```python
from build123d import *

# Parameters (mm, degrees)
F0_W         = 8.5
F0_H         = 13.5
F0_W_2       = 1.7211329822
F0_H_2       = 1.5
F0_W_3       = 1.7788670178
F1_DEPTH     = 0.9
F2_DEPTH     = 1.5
F3_DEPTH     = 7.8
F5_W         = 12
F5_H         = 15
F6_DEPTH     = 1.5
F7_R         = 3
F8_DEPTH     = 16.501
F9_T1_DEPTH  = 5.3
F9_T3_DEPTH  = 8
F9_T5_DEPTH  = 18
F9_T7_DEPTH  = 21
F9_S11_W     = 2
F9_S11_H     = 2
F9_T12_DEPTH = 2
F9_S17_W     = 2
F9_S17_H     = 2
F9_T18_DEPTH = 2
F9_S23_W     = 2
F9_S23_H     = 2
F9_T24_DEPTH = 2
F9_S29_W     = 2
F9_S29_H     = 2
F9_T30_DEPTH = 2


# Not quite as in the source:
# - a fillet or chamfer that OpenCascade refuses, or shapes differently, is made with other operations: its cross-section is extruded or revolved along the edge and cut away or added
# - a feature names something its author has since deleted; it is built from what else it names


with BuildPart() as f1:
    # F0 (on Top) → F1 (new body)
    with BuildSketch(Plane.XY):
        with Locations((-0.0288670178, 8.25)):
            Rectangle(F0_W, F0_H)
        Polygon((-6, 1.5), (-6, -1.5), (-4.2211329822, -1.5), (-4.2413398946, -0.45), (-5.25, -0.45), (-5.25, 0.45), (-4.2586601054, 0.45), (-4.2788670178, 1.5), align=None)
        Polygon((4.2211329822, 1.5), (-4.2788670178, 1.5), (-4.2586601054, 0.45), (4.2413398946, 0.45), align=None)
        with Locations((-5.1394335089, 8.25)):
            Rectangle(F0_W_2, F0_H)
        Polygon((4.2586601054, -0.45), (4.2788670178, -1.5), (6, -1.5), (6, 1.5), (4.2211329822, 1.5), (4.2413398946, 0.45), (5.25, 0.45), (5.25, -0.45), align=None)
        Polygon((-4.2413398946, -0.45), (-4.2211329822, -1.5), (4.2788670178, -1.5), (4.2586601054, -0.45), align=None)
        Polygon((-4.2586601054, 0.45), (-4.2413398946, -0.45), (4.2586601054, -0.45), (4.2413398946, 0.45), align=None)
        Polygon((-5.25, -0.45), (-4.2413398946, -0.45), (-4.2586601054, 0.45), (-5.25, 0.45), align=None)
        Polygon((4.2413398946, 0.45), (4.2586601054, -0.45), (5.25, -0.45), (5.25, 0.45), align=None)
        with Locations((-5.1394335089, 15.75)):
            Rectangle(F0_W_2, F0_H_2)
        with Locations((-0.0288670178, 15.75)):
            Rectangle(F0_W, F0_H_2)
        with Locations((5.1105664911, 15.75)):
            Rectangle(F0_W_3, F0_H_2)
        with Locations((5.1105664911, 8.25)):
            Rectangle(F0_W_3, F0_H)
    extrude(amount=F1_DEPTH)

    # F0 (on Top) → F2 (join)
    with BuildSketch(Plane.XY):
        Polygon((-4.2413398946, -0.45), (-4.2211329822, -1.5), (4.2788670178, -1.5), (4.2586601054, -0.45), align=None)
        Polygon((-6, 1.5), (-6, -1.5), (-4.2211329822, -1.5), (-4.2413398946, -0.45), (-5.25, -0.45), (-5.25, 0.45), (-4.2586601054, 0.45), (-4.2788670178, 1.5), align=None)
        Polygon((4.2586601054, -0.45), (4.2788670178, -1.5), (6, -1.5), (6, 1.5), (4.2211329822, 1.5), (4.2413398946, 0.45), (5.25, 0.45), (5.25, -0.45), align=None)
        Polygon((4.2211329822, 1.5), (-4.2788670178, 1.5), (-4.2586601054, 0.45), (4.2413398946, 0.45), align=None)
        with Locations((-5.1394335089, 8.25)):
            Rectangle(F0_W_2, F0_H)
        with Locations((5.1105664911, 8.25)):
            Rectangle(F0_W_3, F0_H)
        with Locations((-0.0288670178, 8.25)):
            Rectangle(F0_W, F0_H)
        with Locations((-5.1394335089, 15.75)):
            Rectangle(F0_W_2, F0_H_2)
        with Locations((-0.0288670178, 15.75)):
            Rectangle(F0_W, F0_H_2)
        with Locations((5.1105664911, 15.75)):
            Rectangle(F0_W_3, F0_H_2)
    extrude(amount=F2_DEPTH)

    # F0 (on Top) → F3 (join)
    with BuildSketch(Plane.XY):
        Polygon((-6, 1.5), (-6, -1.5), (-4.2211329822, -1.5), (-4.2413398946, -0.45), (-5.25, -0.45), (-5.25, 0.45), (-4.2586601054, 0.45), (-4.2788670178, 1.5), align=None)
        Polygon((4.2586601054, -0.45), (4.2788670178, -1.5), (6, -1.5), (6, 1.5), (4.2211329822, 1.5), (4.2413398946, 0.45), (5.25, 0.45), (5.25, -0.45), align=None)
        with Locations((-5.1394335089, 8.25)):
            Rectangle(F0_W_2, F0_H)
        with Locations((5.1105664911, 8.25)):
            Rectangle(F0_W_3, F0_H)
        with Locations((-5.1394335089, 15.75)):
            Rectangle(F0_W_2, F0_H_2)
        with Locations((-0.0288670178, 15.75)):
            Rectangle(F0_W, F0_H_2)
        with Locations((5.1105664911, 15.75)):
            Rectangle(F0_W_3, F0_H_2)
    extrude(amount=F3_DEPTH)

    # F5 (on offset) → F6 (join)
    with BuildSketch(Plane.XY.offset(7.8)):
        with Locations((0, 9)):
            Rectangle(F5_W, F5_H)
    extrude(amount=F6_DEPTH)

    # F7 (on Front) → F8 (cut, through all)
    with BuildSketch(Plane.XZ):
        with Locations((0, 4.5)):
            Circle(F7_R)
    extrude(amount=-F8_DEPTH, mode=Mode.SUBTRACT)

    # F9: fillet of radius 2 on 8 edges, made by hand

    # F9_s2 → F9_t1 (cut)
    with BuildSketch(Plane.XY.offset(2)):
        with BuildLine():
            ThreePointArc((4, 16.5), (5.4142135624, 15.9142135624), (6, 14.5))
            Line((6, 14.5), (6, 16.5))
            Line((6, 16.5), (4, 16.5))
        make_face()
        with BuildLine():
            ThreePointArc((-4, 16.5), (-5.4142135624, 15.9142135624), (-6, 14.5))
            Line((-6, 14.5), (-6, 16.5))
            Line((-6, 16.5), (-4, 16.5))
        make_face()
    extrude(amount=F9_T1_DEPTH, mode=Mode.SUBTRACT)

    # F9_s4 → F9_t3 (cut)
    with BuildSketch(Plane.YZ.offset(-4)):
        with BuildLine():
            ThreePointArc((16.5, 7.3), (15.9142135624, 8.7142135624), (14.5, 9.3))
            Line((14.5, 9.3), (16.5, 9.3))
            Line((16.5, 9.3), (16.5, 7.3))
        make_face()
        with BuildLine():
            ThreePointArc((14.5, 0), (15.9142135624, 0.5857864376), (16.5, 2))
            Line((16.5, 2), (16.5, 0))
            Line((16.5, 0), (14.5, 0))
        make_face()
    extrude(amount=F9_T3_DEPTH, mode=Mode.SUBTRACT)

    # F9_s6 → F9_t5 (cut)
    with BuildSketch(Plane.XZ.offset(-14.5)):
        with BuildLine():
            ThreePointArc((4, 9.3), (5.4142135624, 8.7142135624), (6, 7.3))
            Line((6, 7.3), (6, 9.3))
            Line((6, 9.3), (4, 9.3))
        make_face()
        with BuildLine():
            ThreePointArc((-4, 9.3), (-5.4142135624, 8.7142135624), (-6, 7.3))
            Line((-6, 7.3), (-6, 9.3))
            Line((-6, 9.3), (-4, 9.3))
        make_face()
    extrude(amount=F9_T5_DEPTH, mode=Mode.SUBTRACT)

    # F9_s8 → F9_t7 (cut)
    with BuildSketch(Plane.XZ.offset(-14.5)):
        with BuildLine():
            ThreePointArc((4, 0), (5.4142135624, 0.5857864376), (6, 2))
            Line((6, 2), (6, 0))
            Line((6, 0), (4, 0))
        make_face()
        with BuildLine():
            ThreePointArc((-4, 0), (-5.4142135624, 0.5857864376), (-6, 2))
            Line((-6, 2), (-6, 0))
            Line((-6, 0), (-4, 0))
        make_face()
    extrude(amount=F9_T7_DEPTH, mode=Mode.SUBTRACT)


with BuildPart() as f9_tool10:
    # F9_s11 → F9_t12 (new body)
    with BuildSketch(Plane.XY.offset(2)):
        with Locations((5, 15.5)):
            Rectangle(F9_S11_W, F9_S11_H)
    extrude(amount=-F9_T12_DEPTH)

    # F9_s13 → F9_t14 (revolve, cut)
    with BuildSketch(Plane(origin=(4, 14.5, 2), x_dir=(-0.7071067812, -0.7071067812, 0), z_dir=(0.7071067812, -0.7071067812, 0))):
        with BuildLine():
            ThreePointArc((0, -2), (2, 0), (0, 2))
            Line((0, 2), (0, -2))
        make_face()
    revolve(axis=Axis((4, 14.5, 2), (0, 0, -1)), mode=Mode.SUBTRACT)


with BuildPart() as f1_1:
    add(f1.part)

    # F9_t9: cut F9_tool10
    add(f9_tool10.part, mode=Mode.SUBTRACT)


with BuildPart() as f9_tool16:
    # F9_s17 → F9_t18 (new body)
    with BuildSketch(Plane.XY.offset(7.3)):
        with Locations((5, 15.5)):
            Rectangle(F9_S17_W, F9_S17_H)
    extrude(amount=F9_T18_DEPTH)

    # F9_s19 → F9_t20 (revolve, cut)
    with BuildSketch(Plane(origin=(4, 14.5, 7.3), x_dir=(-0.7071067812, -0.7071067812, 0), z_dir=(-0.7071067812, 0.7071067812, 0))):
        with BuildLine():
            ThreePointArc((0, -2), (2, 0), (0, 2))
            Line((0, 2), (0, -2))
        make_face()
    revolve(axis=Axis((4, 14.5, 7.3), (0, 0, 1)), mode=Mode.SUBTRACT)


with BuildPart() as f1_2:
    add(f1_1.part)

    # F9_t15: cut F9_tool16
    add(f9_tool16.part, mode=Mode.SUBTRACT)


with BuildPart() as f9_tool22:
    # F9_s23 → F9_t24 (new body)
    with BuildSketch(Plane.YZ.offset(-4)):
        with Locations((15.5, 8.3)):
            Rectangle(F9_S23_W, F9_S23_H)
    extrude(amount=-F9_T24_DEPTH)

    # F9_s25 → F9_t26 (revolve, cut)
    with BuildSketch(Plane(origin=(-4, 14.5, 7.3), x_dir=(0, -0.7071067812, -0.7071067812), z_dir=(0, 0.7071067812, -0.7071067812))):
        with BuildLine():
            ThreePointArc((0, -2), (2, 0), (0, 2))
            Line((0, 2), (0, -2))
        make_face()
    revolve(axis=Axis((-4, 14.5, 7.3), (-1, 0, 0)), mode=Mode.SUBTRACT)


with BuildPart() as f1_3:
    add(f1_2.part)

    # F9_t21: cut F9_tool22
    add(f9_tool22.part, mode=Mode.SUBTRACT)


with BuildPart() as f9_tool28:
    # F9_s29 → F9_t30 (new body)
    with BuildSketch(Plane.YZ.offset(-4)):
        with Locations((15.5, 1)):
            Rectangle(F9_S29_W, F9_S29_H)
    extrude(amount=-F9_T30_DEPTH)

    # F9_s31 → F9_t32 (revolve, cut)
    with BuildSketch(Plane(origin=(-4, 14.5, 2), x_dir=(0, -0.7071067812, 0.7071067812), z_dir=(0, -0.7071067812, -0.7071067812))):
        with BuildLine():
            ThreePointArc((0, -2), (2, 0), (0, 2))
            Line((0, 2), (0, -2))
        make_face()
    revolve(axis=Axis((-4, 14.5, 2), (-1, 0, 0)), mode=Mode.SUBTRACT)


with BuildPart() as f1_4:
    add(f1_3.part)

    # F9_t27: cut F9_tool28
    add(f9_tool28.part, mode=Mode.SUBTRACT)


solid = f1_4.part
```
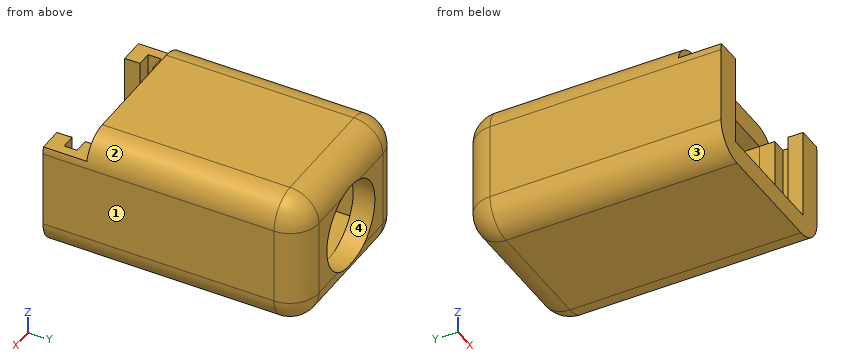
Build history of the part. All positions in model axes, mm. Face numbers are marked on the shaded views. Round coordinates to 2 decimals unless told otherwise and drop trailing zeros. Loops run counter-clockwise (first coordinate to the right, second up) from the corner with the lowest first, then second, coordinate; pieces in that order, holes last. Notation, with made-up numbers: M 41,73 L 59,73 A29 ccw 59,107 Z; hole C 14,87 d2. An arc over 180 degrees is marked long. Answer as CSV lines item,"result".
1. Cut at B-B on y = 7.75. Write the cut outline in (x, z), then the cut area to 3 significant figures.
Resolved:
outline,"M -6,2 A2 ccw -4,0 L 4,0 A2 ccw 6,2 L 6,7.3 A2 ccw 4,9.3 L -4,9.3 A2 ccw -6,7.3 Z; hole M -4.28,1.5 L 4.22,1.5 L 4.22,7.8 L -4.28,7.8 Z"
area,"54.6 mm²"
2. Two-plate mould, pull along Z, no slides. Class the marked faces 1, 2, 3 and 4: released by +Z, released by -Z, zero draft, split by the parting line, or undercut.
Resolved:
face 1,"zero draft"
face 2,"released by +Z"
face 3,"released by -Z"
face 4,"undercut"
3. Wall check: probe 1 along X at (y, z) = (-0.5, 2.5); probe 2 along Z at (x, y) = (-2, 13.5); probe 3 along X at (y, z) = (-0.25, 3). Give the ranges that are in metal, low to high. Write a range as [from, to].
Resolved:
probe 1,"x = [-6, -4.24], [4.26, 6]"
probe 2,"z = [0, 1.5], [7.8, 9.3]"
probe 3,"x = [-6, -5.25], [5.25, 6]"
4. Flat gauge pins, fed straight in: P1, Ø1, axis at x = 0, y = 0, coming from the +Z side; P2, Ø3.5, axis at x = 0, z = 4.5, coming from the +Y side; P3, Ø0.8, axis at x = -0.5, z = 8.5, coming from the -Y side; P4, Ø1.9, axis at x = -5, y = 0.5, coming from the +Z side. Where does each tip first touch, or does it go through?
Resolved:
P1,"stops at z = 1.5"
P2,"passes through"
P3,"stops at y = 1.5"
P4,"stops at z = 7.8"
5. Cut at D-D on x = -4.75. Write the cut outline in (y, z).
Resolved:
outline,"M -1.5,0.15 L 14.5,0.15 A1.85 ccw 16.35,2 L 16.35,7.3 A1.85 ccw 14.5,9.15 L 1.5,9.15 L 1.5,7.8 L 0.45,7.8 L 0.45,0.9 L -0.45,0.9 L -0.45,7.8 L -1.5,7.8 Z"
6. Cut at C-C on z = 1.25. Write the cut outline in (x, y), then the cut area to 3 significant figures.
Resolved:
outline,"M -5.85,-1.5 L 5.85,-1.5 L 5.85,14.5 A1.85 ccw 4,16.35 L -4,16.35 A1.85 ccw -5.85,14.5 Z; hole M -5.25,-0.45 L 5.25,-0.45 L 5.25,0.45 L -5.25,0.45 Z"
area,"198 mm²"
7. Cut at A-A on z = 4.5. Write the cut outline in (x, y).
Resolved:
outline,"M -6,-1.5 L -4.22,-1.5 L -4.24,-0.45 L -5.25,-0.45 L -5.25,0.45 L -4.26,0.45 L -4.28,1.5 L -4.28,15 L -3,15 L -3,16.5 L -4,16.5 A2 ccw -6,14.5 Z; M 3,15 L 4.22,15 L 4.22,1.5 L 4.24,0.45 L 5.25,0.45 L 5.25,-0.45 L 4.26,-0.45 L 4.28,-1.5 L 6,-1.5 L 6,14.5 A2 ccw 4,16.5 L 3,16.5 Z"
